The drawing under review shows one solid part. Ordinate dimensions are in mm from its lowest x, y, z. Give positions to 0.01 mm unless a question says otherwise; leave off trailing zeros. Loops run counter-clockwise (first coordinate to the right, second up) from the corner with the lowest first, then second, coordinate; pieces in that order, holes last. Notation, with made-up numbers: (63.25, 87.25) - (82.25, 87.25) arc R34 cw to (82.25, 118.25) - close; hole circle Ø9 at (88.5, -38). An arc over 180 degrees is marked (long way). Answer as CSV lines item,"result".
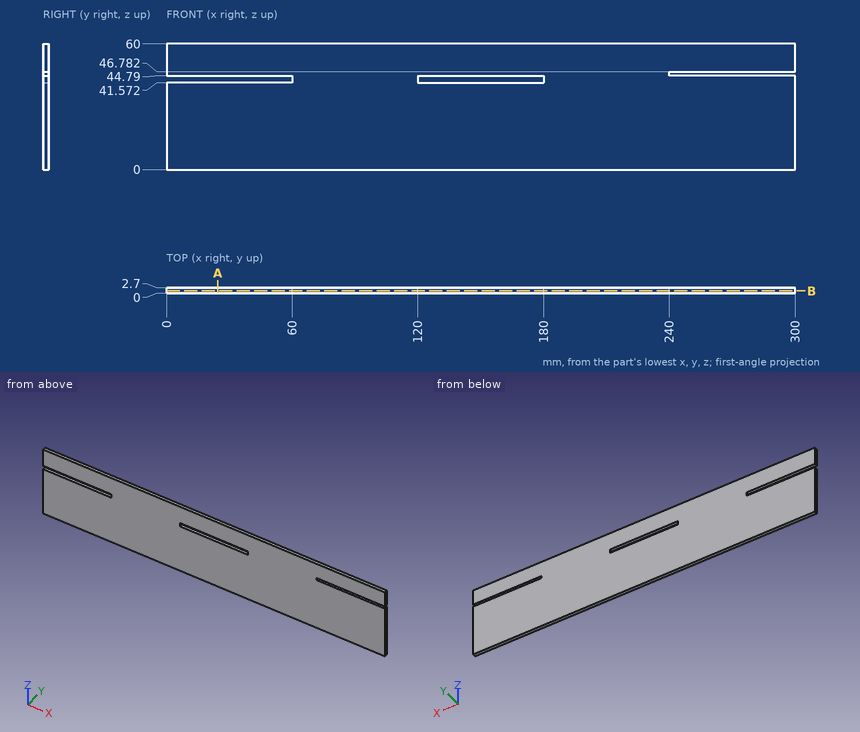
1) Consider section B-B on y = 1.15. Write out the cut boundary in (x, z).
From the geometry:
outline,"(0, 0) - (300, 0) - (300, 44.79) - (240, 44.79) - (240, 46.78) - (300, 46.78) - (300, 60) - (0, 60) - (0, 44.79) - (60, 44.79) - (60, 41.57) - (0, 41.57) - close; hole (120, 41.57) - (180, 41.57) - (180, 44.79) - (120, 44.79) - close"
2) Consider section A-A on x = 24.5. Write out the cut boundary in (y, z).
From the geometry:
outline,"(0, 0) - (2.7, 0) - (2.7, 41.57) - (0, 41.57) - close; (0, 44.79) - (2.7, 44.79) - (2.7, 60) - (0, 60) - close"
3) Wall thickness on line 1 (Z direction, x = 259, y = 0.1); line 2 (Z direction, x = 169, y = 0.55): over which ranges is each line inside the solid? List them lowest first. Write a range as from..to.
From the geometry:
line 1,"z = 0..44.79, 46.78..60"
line 2,"z = 0..41.57, 44.79..60"
4) Insertion check: P1, Ø0.8, axis at y = 1, z = 43, coming from the -X side; P2, Ø1, axis at y = 1.5, z = 46, coming from the +X side. Each pin has a flat end and moves straight along its axis. Give the tip position at first contact, or say it passes through.
From the geometry:
P1,"stops at x = 60"
P2,"stops at x = 240"
